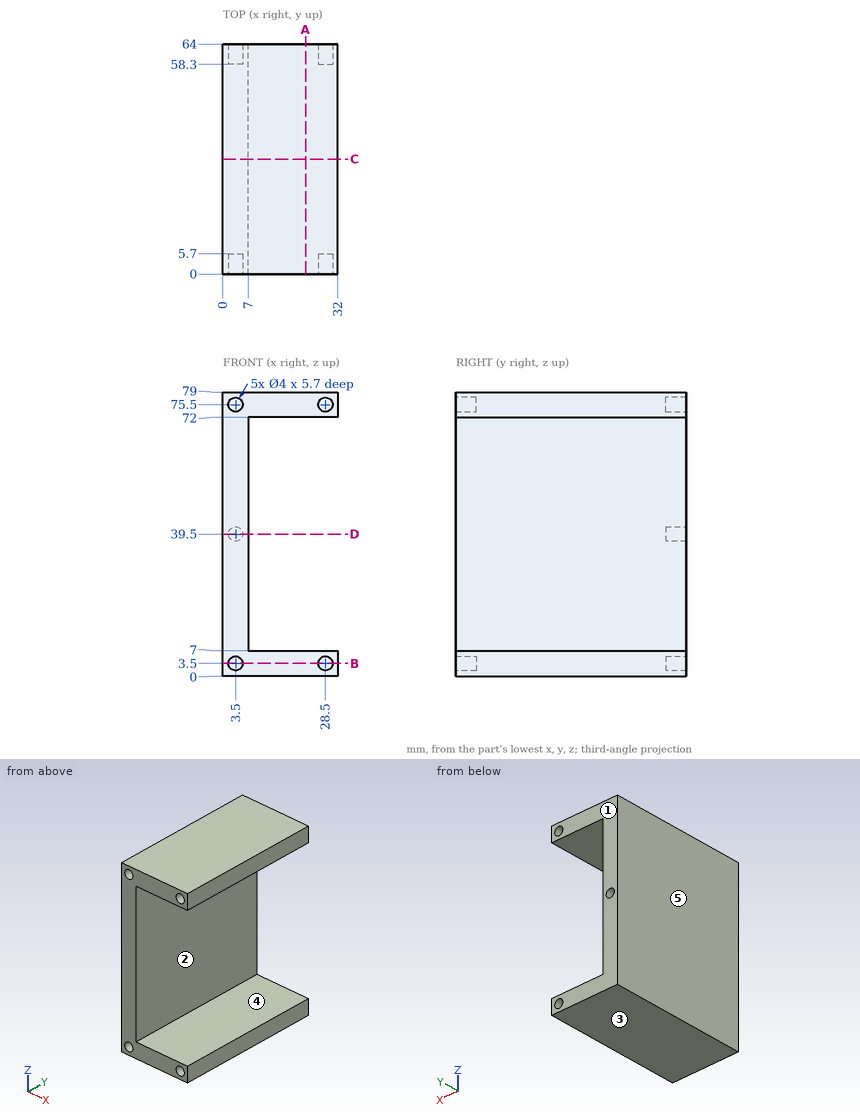
Study the drawing (mm; zero at the part's minimum x, y, z) and answer. A direction names the side the tool comes from. Coordinates: 2 decimals unless noted, no trailing zeros. Loops run counter-clockwise (first coordinate to the right, second up) from the corner with the lowest first, then second, coordinate; pieces in that order, holes last. Notation, with made-up numbers: (6, 16) -> (39, 16) arc R18 ccw to (39, 33) -> close; hole circle Ø6 at (22.5, 56.25). An arc over 180 degrees is marked (long way). Answer as CSV lines item,"result".
1) Flat-ended cylindrical pins translate along their axes: pin 1 (6.5 mm diameter, centred on x = 3.5, z = 3.5, fed in from -Y); pin 2 (2 mm diameter, centred on y = 24.5, z = 30, fed in from +X); pin 3 (1.2 mm diameter, centred on x = 4, z = 74.5, fed in from -Y); pin 4 (1.2 mm diameter, centred on x = 4.5, z = 39.5, fed in from +Y). Find the tip coordinate at first contact, or state that the pin passes through.
A:
pin 1,"stops at y = 0"
pin 2,"stops at x = 7"
pin 3,"stops at y = 5.7"
pin 4,"stops at y = 58.3"
2) The part is cut by section B-B (z = 3.5). Give the vertices of the cut face in (x, y).
A:
outline,"(0, 0) -> (1.5, 0) -> (1.5, 5.7) -> (5.5, 5.7) -> (5.5, 0) -> (26.5, 0) -> (26.5, 5.7) -> (30.5, 5.7) -> (30.5, 0) -> (32, 0) -> (32, 64) -> (30.5, 64) -> (30.5, 58.3) -> (26.5, 58.3) -> (26.5, 64) -> (0, 64) -> close"
3) For the marked faces 1 and 2, determine the directions among +Z, -Z, +X, -X, +Y, -Y from which every point of the face is accessible in a straight line to the end or side of a thin tool.
A:
face 1,"+Z, -Z, +X, -X, +Y"
face 2,"+X, +Y, -Y"
4) The part is cut by section D-D (z = 39.5). Give the vertices of the cut face in (x, y).
A:
outline,"(0, 0) -> (7, 0) -> (7, 64) -> (5.5, 64) -> (5.5, 58.3) -> (1.5, 58.3) -> (1.5, 64) -> (0, 64) -> close"
5) For a pull along Z with two mould halves and no side action, classify the marked faces 3, 4 and 5 as released by +Z, released by -Z, zero draft, split by the parting line, or undercut.
A:
face 3,"released by -Z"
face 4,"undercut"
face 5,"zero draft"
6) The part is cut by section C-C (y = 32). Give the vertices of the cut face in (x, z), and give its area (3 significant figures).
A:
outline,"(0, 0) -> (32, 0) -> (32, 7) -> (7, 7) -> (7, 72) -> (32, 72) -> (32, 79) -> (0, 79) -> close"
area,"903 mm²"
7) Straight lines are drawn through the part: probe 1 along X at (y, z) = (2.5, 75.5); probe 2 along Z at (x, y) = (11.5, 5.5); probe 3 along X at (y, z) = (1, 3). For each, find the intervals that lie inside material, in ascending order.
A:
probe 1,"x = 0 to 1.5, 5.5 to 26.5, 30.5 to 32"
probe 2,"z = 0 to 7, 72 to 79"
probe 3,"x = 0 to 1.56, 5.44 to 26.56, 30.44 to 32"
8) The part is cut by section A-A (x = 23). Give the vertices of the cut face in (y, z), and give its area (3 significant figures).
A:
outline,"(0, 0) -> (64, 0) -> (64, 7) -> (0, 7) -> close; (0, 72) -> (64, 72) -> (64, 79) -> (0, 79) -> close"
area,"896 mm²"
